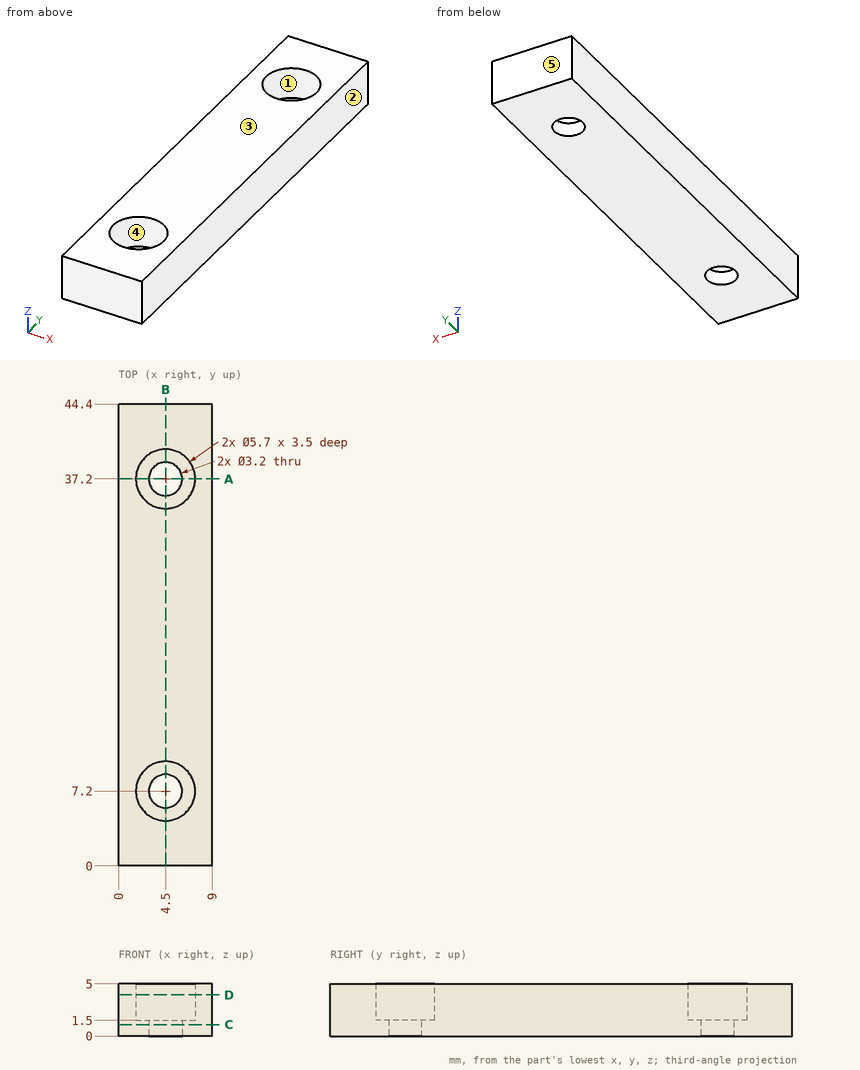
Drawing for the job (mm, zero at the part's lowest x, y, z). A direction names the side the tool comes from. Round coordinates to 2 decimals unless told otherwise and drop trailing zeros. Write each loop counter-clockwise with the first axis right and the second up, starting at its lowest first coordinate (ties: lowest second). Pieces come first, ordered by that corner, then holes. Notation, with made-up numbers: M 53,-5 L 88,-5 A17 ccw 88,10 Z; hole C -37.5,42 d2. An arc over 180 degrees is marked long. One line per question, with ' | ' between items.
1. Which spindle directions (+Z, -Z, +X, -X, +Y, -Y) get a long thin tool onto all of the face, cutting with end or side? Do the marked faces 4 and 5. Say none if no direction does.
Working result:
face 4: +Z | face 5: +Z, -Z, +X, -X, +Y
2. Probe L1, parallel to Y at x = 4.5, z = 0.75; L2, parallel to X at y = 7.2, z = 1; L3, parallel to Y at x = 4.5, z = 4.1. List the from-to ranges inside material, lowest first. Write a range as from..to.
Working result:
L1: 0..5.6, 8.8..35.6, 38.8..44.4 | L2: 0..2.9, 6.1..9 | L3: 0..4.35, 10.05..34.35, 40.05..44.4
3. Mould opens along X. For the marked faces 1, 2 and 3 say: pulls with the +X half, pulls with the -X half, needs draft (parallel to the pull), parting line crosses it, or undercut.
Working result:
face 1: undercut | face 2: pulls with the +X half | face 3: needs draft
4. Cut at A-A on y = 37.2. Write the cut outline in (x, z).
Working result:
outline: M 0,0 L 2.9,0 L 2.9,1.5 L 1.65,1.5 L 1.65,5 L 0,5 Z; M 6.1,0 L 9,0 L 9,5 L 7.35,5 L 7.35,1.5 L 6.1,1.5 Z
5. Cut at B-B on x = 4.5. Write the cut outline in (y, z).
Working result:
outline: M 0,0 L 5.6,0 L 5.6,1.5 L 4.35,1.5 L 4.35,5 L 0,5 Z; M 8.8,0 L 35.6,0 L 35.6,1.5 L 34.35,1.5 L 34.35,5 L 10.05,5 L 10.05,1.5 L 8.8,1.5 Z; M 38.8,0 L 44.4,0 L 44.4,5 L 40.05,5 L 40.05,1.5 L 38.8,1.5 Z
6. Pin check, flat tip, straight feed: pin 1 Ø3.5 at (x, y) = (4.5, 7.2) entering from +Z. Stop position of the tip, or through.
Working result:
pin 1: z = 1.5
7. Cut at C-C on z = 1.1. Write the cut outline in (x, y).
Working result:
outline: M 0,0 L 9,0 L 9,44.4 L 0,44.4 Z; hole C 4.5,7.2 d3.2; hole C 4.5,37.2 d3.2
8. Cut at D-D on z = 3.95. Write the cut outline in (x, y).
Working result:
outline: M 0,0 L 9,0 L 9,44.4 L 0,44.4 Z; hole C 4.5,7.2 d5.7; hole C 4.5,37.2 d5.7
